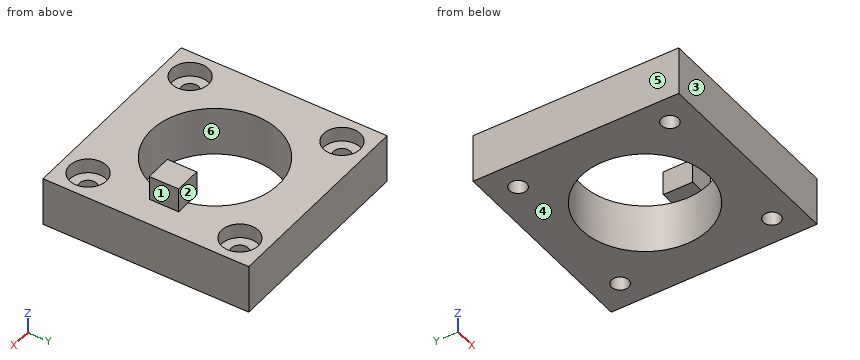
Autodesk Inventor part; units mm, degrees
ref_plane "YZ Plane" through (0, 0, 0) normal (1, 0, 0) x (0, 1, 0)
ref_plane "XZ Plane" through (0, 0, 0) normal (0, 1, 0) x (-1, 0, 0)
ref_plane "XY Plane" through (0, 0, 0) normal (0, 0, 1) x (1, 0, 0)
sketch "Sketch1" plane through (0, 0, 0) normal (0, 0, 1) x (1, 0, 0)
  line L0 (-21, -21) -> (21, -21)
  line L1 (21, -21) -> (21, 21)
  line L2 (21, 21) -> (-21, 21)
  line L3 (-21, 21) -> (-21, -21)
  line L4 (-21, 0) -> (21, 0)
  line L5 (21, 0) -> (19, 0)
  line L6 (0, -21) -> (0, 21)
  point P0 (0, 0)
  point P1 (0, 0)
  dimension "d0" = 42
  dimension "d1" = 42
extrude "Extrusion1" add sketch "Sketch1" along normal blind 10
sketch "Sketch2" plane through (0, 0, 10) normal (0, 0, 1) x (1, 0, 0)
  circle A0 centre (0, 0) radius 13
  circle A1 centre (-15.5, 15.5) radius 1.75
  circle A2 centre (15.5, 15.5) radius 1.75
  circle A3 centre (15.5, -15.5) radius 1.75
  circle A4 centre (-15.5, -15.5) radius 1.75
  line L0 (21, 21) -> (-21, 21)
  line L1 (-21, 21) -> (-21, -21)
  line L2 (-21, -21) -> (21, -21)
  line L3 (21, -21) -> (21, 21)
  line L4 (0, -21) -> (0, 21)
  line L5 (-21, 0) -> (21, 0)
  dimension "d5" = 26
  dimension "d6" = 3.5
  dimension "d7" = 31
  dimension "d8" = 31
extrude "Extrusion2" cut sketch "Sketch2" against normal through all contours L5 L4 A0 | A0 L4 L5 | L4 L5 A0 | A0 L5 L4 | A1 | A2 | A3 | A4
sketch "Sketch3" plane through (0, 0, 10) normal (0, 0, 1) x (1, 0, 0)
  circle A0 centre (15.5, -15.5) radius 1.75
  circle A1 centre (-15.5, -15.5) radius 1.75
  circle A2 centre (0, 0) radius 13
  circle A3 centre (-15.5, 15.5) radius 1.75
  circle A4 centre (15.5, 15.5) radius 1.75
  line L0 (-21, 21) -> (-21, -21)
  line L1 (-21, -21) -> (21, -21)
  line L2 (21, -21) -> (21, 21)
  line L3 (21, 21) -> (-21, 21)
  circle A5 centre (15.5, -15.5) radius 3.75
  circle A6 centre (-15.5, -15.5) radius 3.75
  circle A7 centre (-15.5, 15.5) radius 3.75
  circle A8 centre (15.5, 15.5) radius 3.75
  dimension "d14" = 2
  dimension "d17" = 2
  dimension "d18" = 2
  dimension "d19" = 2
extrude "Extrusion4" cut sketch "Sketch3" against normal blind 3 contours A5 | A6 | A7 | A8
sketch "Sketch5" plane through (0, 0, 10) normal (0, 0, 1) x (1, 0, 0)
  circle A0 centre (-15.5, 15.5) radius 3.75
  circle A1 centre (15.5, -15.5) radius 3.75
  circle A2 centre (-15.5, -15.5) radius 3.75
  circle A3 centre (15.5, 15.5) radius 3.75
  circle A4 centre (0, 0) radius 13
  line L0 (21, 21) -> (-21, 21)
  line L1 (-21, 21) -> (-21, -21)
  line L2 (-21, -21) -> (21, -21)
  line L3 (21, -21) -> (21, 21)
  line L4 (21, -21) -> (21, 21)
  line L5 (21, 0) -> (13, 0)
  line L6 (15.5, 3) -> (15.5, -3)
  line L7 (15.5, 3) -> (10, 3)
  line L8 (10, 3) -> (10, -3)
  line L9 (10, -3) -> (15.5, -3)
  dimension "d27" = 6
extrude "Extrusion5" add sketch "Sketch5" along normal blind 5 contours A4 L9 L8 L7 | L5 L6 L9 A4 | A4 L7 L6 L5 picked at (11, 0)
properties part number "soporte02"
Can you work these out from the model? Positions are in its coordinate system, mm. Face numbers are marked on the shaded views. A direction names the side the tool comes from. Coordinates: 2 decimals unless noted, no trailing zeros. Loops run counter-clockwise (first coordinate to the right, second up) from the corner with the lowest first, then second, coordinate; pieces in that order, holes last. Notation, with made-up numbers: M -40,32.25 L -34,32.25 A17 cw -34,36.25 Z; hole C 11.25,-36 d11. An arc over 180 degrees is marked long. Return JSON: item names as keys, results as strings. Group by question number.
Item 1: Imagine slicing it at C-C (x = 0). Please give me the cut outline in (y, z), and give its area (3 significant figures).
Item 2: Thinking about a two-plate mould opening in X: for the marked faces 4, 5 and 6, which applies, released by +X, released by -X, zero draft, split by the parting line, or undercut?
Item 3: I'm going to push flat-ended pins straight in: pin 1 Ø4 at (y, z) = (0, 13.5) entering from -X; pin 2 Ø4 at (x, y) = (14.5, 17) entering from +Z; pin 3 Ø2 at (x, y) = (-14, 16.5) entering from +Z; pin 4 Ø3 at (x, y) = (-15.5, 15.5) entering from +Z. Where does each tip first touch, or does it pass through?
Item 4: Imagine slicing it at D-D (y = 0). Please give me the cut outline in (x, z), and give its area (4 significant figures).
Item 5: Imagine slicing it at A-A (x = -15.5). Please give me the cut outline in (y, z), and give its area (3 significant figures).
Item 6: If I drill on L1, parallel to Y at x = 15.5, z = 8.3; L2, parallel to Y at x = 0, z = 8; L3, parallel to Y at x = -14, z = 2.5, over which ranges is the centre line in solid material (lowest first)? Write a range as from..to.
Item 7: On a 3-axis mill with a long thin cutter (end or side, diameter ignored), from which of +Z, -Z, +X, -X, +Y, -Y can I reach the whole of each face in a straight line? I mean the marked faces 1, 2 and 3. Say none if no direction works.
Verdict:
{
 "1": {"outline": "M -21,0 L -13,0 L -13,10 L -21,10 Z; M 13,0 L 21,0 L 21,10 L 13,10 Z", "area": "160 mm^2"},
 "2": {"face 4": "zero draft", "face 5": "released by -X", "face 6": "undercut"},
 "3": {"pin 1": "stops at x = 10", "pin 2": "stops at z = 10", "pin 3": "stops at z = 7", "pin 4": "passes through"},
 "4": {"outline": "M -21,0 L -13,0 L -13,10 L -21,10 Z; M 10,10 L 13,10 L 13,0 L 21,0 L 21,10 L 15.5,10 L 15.5,15 L 10,15 Z", "area": "187.5 mm^2"},
 "5": {"outline": "M -21,0 L -17.25,0 L -17.25,7 L -19.25,7 L -19.25,10 L -21,10 Z; M -13.75,0 L 13.75,0 L 13.75,7 L 11.75,7 L 11.75,10 L -11.75,10 L -11.75,7 L -13.75,7 Z; M 17.25,0 L 21,0 L 21,10 L 19.25,10 L 19.25,7 L 17.25,7 Z", "area": "326 mm^2"},
 "6": {"L1": "y = -21..-19.25, -11.75..11.75, 19.25..21", "L2": "y = -21..-13, 13..21", "L3": "y = -21..-16.4, -14.6..14.6, 16.4..21"},
 "7": {"face 1": "+Z, +X, +Y, -Y", "face 2": "+Z, +X, -X, +Y", "face 3": "+Z, -Z, +X, -X, -Y"}
}
